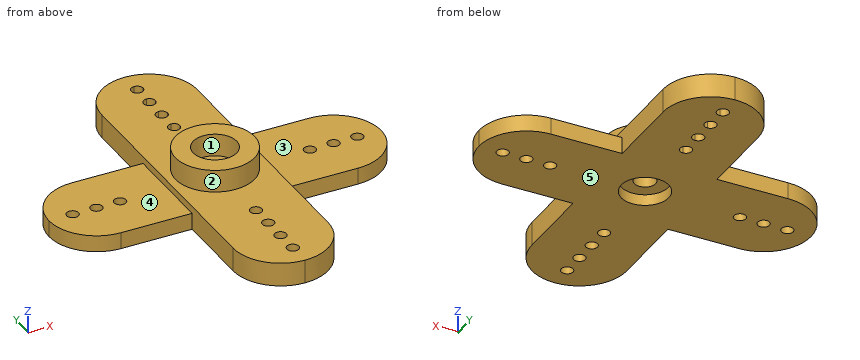
from build123d import *

# Parameters (mm, degrees)
F0_R     = 19.05
F1_DEPTH = 76.2
F2_DEPTH = 53.34
F3_R     = 127
F3_R_2   = 69.85
F4_DEPTH = 72.39
F5_R     = 76.2
F6_DEPTH = 35.56


with BuildPart() as f1:
    # F0 (on Top) → F1 (new body)
    with BuildSketch(Plane.XY):
        with BuildLine():
            ThreePointArc((34.29, 0), (-24.246692, -24.246692), (0, 34.29))
            Line((0, 34.29), (0, 234.95))
            ThreePointArc((0, 234.95), (-19.05, 254), (0, 273.05))
            Line((0, 273.05), (0, 311.15))
            ThreePointArc((0, 311.15), (-19.05, 330.2), (0, 349.25))
            Line((0, 349.25), (0, 387.35))
            ThreePointArc((0, 387.35), (-19.05, 406.4), (0, 425.45))
            Line((0, 425.45), (0, 463.55))
            ThreePointArc((0, 463.55), (-19.05, 482.6), (0, 501.65))
            Line((0, 501.65), (0, 558.8))
            ThreePointArc((0, 558.8), (-107.763073, 514.163073), (-152.4, 406.4))
            Line((-152.4, 406.4), (-152.4, 152.4))
            Line((-152.4, 152.4), (-152.4, -152.4))
            Line((-152.4, -152.4), (-152.4, -406.4))
            ThreePointArc((-152.4, -406.4), (-107.763073, -514.163073), (0, -558.8))
            ThreePointArc((0, -558.8), (107.763073, -514.163073), (152.4, -406.4))
            Line((152.4, -406.4), (152.4, -152.4))
            Line((152.4, -152.4), (152.4, 0))
            Line((152.4, 0), (34.29, 0))
        make_face()
        with Locations((0, -482.6)):
            Circle(F0_R, mode=Mode.SUBTRACT)
        with Locations((0, -406.4)):
            Circle(F0_R, mode=Mode.SUBTRACT)
        with Locations((0, -330.2)):
            Circle(F0_R, mode=Mode.SUBTRACT)
        with Locations((0, -254)):
            Circle(F0_R, mode=Mode.SUBTRACT)
        with BuildLine():
            Line((0, 234.95), (0, 34.29))
            ThreePointArc((0, 34.29), (24.246692, 24.246692), (34.29, 0))
            Line((34.29, 0), (152.4, 0))
            Line((152.4, 0), (152.4, 152.4))
            Line((152.4, 152.4), (152.4, 406.4))
            ThreePointArc((152.4, 406.4), (107.763073, 514.163073), (0, 558.8))
            Line((0, 558.8), (0, 501.65))
            ThreePointArc((0, 501.65), (13.470384, 496.070384), (19.05, 482.6))
            ThreePointArc((19.05, 482.6), (13.470384, 469.129616), (0, 463.55))
            Line((0, 463.55), (0, 425.45))
            ThreePointArc((0, 425.45), (13.470384, 419.870384), (19.05, 406.4))
            ThreePointArc((19.05, 406.4), (13.470384, 392.929616), (0, 387.35))
            Line((0, 387.35), (0, 349.25))
            ThreePointArc((0, 349.25), (13.470384, 343.670384), (19.05, 330.2))
            ThreePointArc((19.05, 330.2), (13.470384, 316.729616), (0, 311.15))
            Line((0, 311.15), (0, 273.05))
            ThreePointArc((0, 273.05), (13.470384, 267.470384), (19.05, 254))
            ThreePointArc((19.05, 254), (13.470384, 240.529616), (0, 234.95))
        make_face()
    extrude(amount=F1_DEPTH)

    # F0 (on Top) → F2 (join)
    with BuildSketch(Plane.XY):
        with BuildLine():
            Line((-381, -152.4), (-152.4, -152.4))
            Line((-152.4, -152.4), (-152.4, 152.4))
            Line((-152.4, 152.4), (-381, 152.4))
            ThreePointArc((-381, 152.4), (-488.763073, 107.763073), (-533.4, 0))
            ThreePointArc((-533.4, 0), (-488.763073, -107.763073), (-381, -152.4))
        make_face()
        with Locations((-457.2, 0)):
            Circle(F0_R, mode=Mode.SUBTRACT)
        with Locations((-381, 0)):
            Circle(F0_R, mode=Mode.SUBTRACT)
        with Locations((-304.8, 0)):
            Circle(F0_R, mode=Mode.SUBTRACT)
        with BuildLine():
            Line((152.4, 152.4), (152.4, 0))
            Line((152.4, 0), (285.75, 0))
            ThreePointArc((285.75, 0), (304.8, 19.05), (323.85, 0))
            Line((323.85, 0), (361.95, 0))
            ThreePointArc((361.95, 0), (381, 19.05), (400.05, 0))
            Line((400.05, 0), (438.15, 0))
            ThreePointArc((438.15, 0), (457.2, 19.05), (476.25, 0))
            Line((476.25, 0), (533.4, 0))
            ThreePointArc((533.4, 0), (488.763073, 107.763073), (381, 152.4))
            Line((381, 152.4), (152.4, 152.4))
        make_face()
        with BuildLine():
            Line((285.75, 0), (152.4, 0))
            Line((152.4, 0), (152.4, -152.4))
            Line((152.4, -152.4), (381, -152.4))
            ThreePointArc((381, -152.4), (488.763073, -107.763073), (533.4, 0))
            Line((533.4, 0), (476.25, 0))
            ThreePointArc((476.25, 0), (457.2, -19.05), (438.15, 0))
            Line((438.15, 0), (400.05, 0))
            ThreePointArc((400.05, 0), (381, -19.05), (361.95, 0))
            Line((361.95, 0), (323.85, 0))
            ThreePointArc((323.85, 0), (304.8, -19.05), (285.75, 0))
        make_face()
    extrude(amount=F2_DEPTH)

    # F3 (on face) → F4 (join)
    with BuildSketch(Plane.XY.offset(76.2)):
        Circle(F3_R)
        Circle(F3_R_2, mode=Mode.SUBTRACT)
    extrude(amount=F4_DEPTH)

    # F5 (on face) → F6 (cut)
    with BuildSketch(Plane.XY):
        Circle(F5_R)
    extrude(amount=F6_DEPTH, mode=Mode.SUBTRACT)


solid = f1.part
Check sheet for the modelled part. Datum: model origin and axes. Units: mm. Face numbers are marked on the shaded views. A direction names the side the tool comes from. Round coordinates to 2 decimals unless told otherwise and drop trailing zeros. Loops run counter-clockwise (first coordinate to the right, second up) from the corner with the lowest first, then second, coordinate; pieces in that order, holes last.
1. Gauge pin test, flat ends, axial feed: pin 1 Ø1.5 at (y, z) = (236.5, 53) entering from -X; pin 2 Ø5 at (x, y) = (207.5, -89.5) entering from +Z; pin 3 Ø16 at (x, z) = (-294, 29.5) entering from +Y. Record the tip position at first contact, or that the pin passes through.
2. Sectioned sample at D-D on x = 96.5. Record the boundary of the cut face in (y, z), and give its area (3 significant figures).
3. Sectioned sample at B-B on y = -254. Record the boundary of the cut face in (x, z), and give its area (3 significant figures).
4. Sectioned sample at C-C on z = 113.5. Record the boundary of the cut face in (x, y).
5. Sectioned sample at A-A on x = -304.8. Record the boundary of the cut face in (y, z).
6. Scan lines: probe 1 along X at (y, z) = (-5.5, 100); probe 2 along Y at (x, z) = (304.8, 21); probe 3 along Y at (x, z) = (224, 45). Record each from-to range of solid material in increasing order.
7. Set-up check for the marked faces 4 and 5: record each of +Z, -Z, +X, -X, +Y, -Y from which the full face is reachable in a straight line by a thin tool's end or side.
8. Mould release check, pull along X, two halves, no side actions. Record for the marked faces 1, 2 and 3: released by +X, released by -X, zero draft, split by the parting line, or undercut.
Recorded:
1. pin 1: stops at x = -152.4
1. pin 2: stops at z = 53.34
1. pin 3: stops at y = 152.4
2. outline: (-524.36, 0) - (524.36, 0) - (524.36, 76.2) - (82.56, 76.2) - (82.56, 148.59) - (-82.56, 148.59) - (-82.56, 76.2) - (-524.36, 76.2) - close
2. area: 91,900 mm2
3. outline: (-152.4, 0) - (-19.05, 0) - (-19.05, 76.2) - (-152.4, 76.2) - close; (19.05, 0) - (152.4, 0) - (152.4, 76.2) - (19.05, 76.2) - close
3. area: 20,300 mm2
4. outline: circle Ø254 at (0, 0); hole circle Ø139.7 at (0, 0)
5. outline: (-152.4, 0) - (-19.05, 0) - (-19.05, 53.34) - (-152.4, 53.34) - close; (19.05, 0) - (152.4, 0) - (152.4, 53.34) - (19.05, 53.34) - close
6. probe 1: x = -126.88 to -69.63, 69.63 to 126.88
6. probe 2: y = -152.4 to -19.05, 19.05 to 152.4
6. probe 3: y = -152.4 to 152.4
7. face 4: +Z, -X, +Y, -Y
7. face 5: -Z, +X, -X, +Y, -Y
8. face 1: undercut
8. face 2: split by the parting line
8. face 3: zero draft
